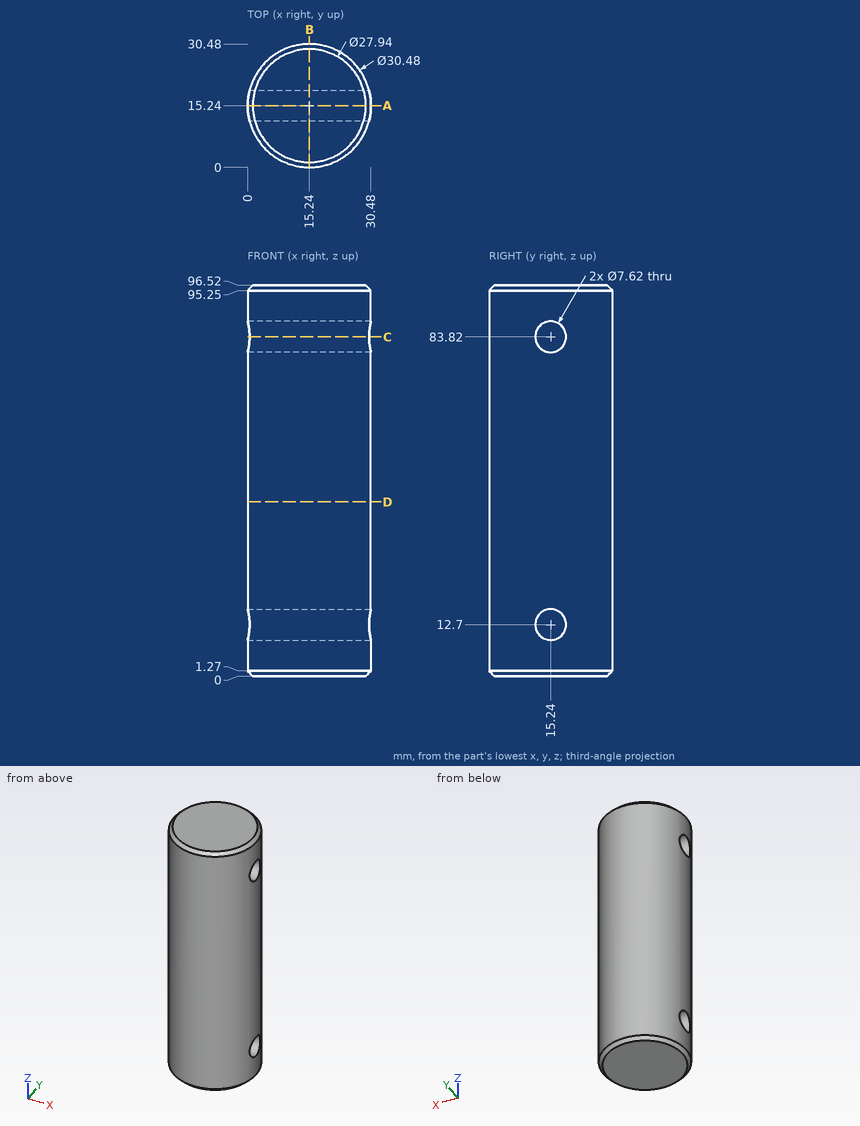
Source: three-view drawing plus pictorial views. Frame: mm from the lowest corner of the part. Coordinates: 2 decimals unless noted, no trailing zeros. Write each loop counter-clockwise with the first axis right and the second up, starting at its lowest first coordinate (ties: lowest second). Pieces come first, ordered by that corner, then holes. Notation, with made-up numbers: (62, 86.5) - (87, 86.5) arc R17 cw to (87, 102.5) - close; hole circle Ø9 at (33, -31). An arc over 180 degrees is marked (long way). Return JSON: item names as keys, results as strings.
Item 1: Pin query (flat end, axial travel): pin 1 Ø1.5 at (x, z) = (7.5, 31.5) entering from -Y; pin 2 Ø8 at (y, z) = (20, 22) entering from +X; pin 3 Ø10 at (y, z) = (15.24, 12.7) entering from -X; pin 4 Ø1.5 at (y, z) = (17, 9.5) entering from +X. Return the tip coordinate at first contact, or that it passes through.
Completed:
{"pin 1": "stops at y = 1.7", "pin 2": "stops at x = 30.46", "pin 3": "stops at x = 0", "pin 4": "stops at x = 30.44"}
Item 2: Section query D-D (z = 43). Output: boundary loops of the cut face in (x, y), and give its area (3 significant figures).
Completed:
{"outline": "circle Ø30.48 at (15.24, 15.24)", "area": "730 mm2"}
Item 3: Section query B-B (x = 15.24). Output: boundary loops of the cut face in (y, z).
Completed:
{"outline": "(0, 1.27) - (1.27, 0) - (29.21, 0) - (30.48, 1.27) - (30.48, 95.25) - (29.21, 96.52) - (1.27, 96.52) - (0, 95.25) - close; hole circle Ø7.62 at (15.24, 12.7); hole circle Ø7.62 at (15.24, 83.82)"}
Item 4: Line query: L1, parallel to Z at x = 19, y = 15; L2, parallel to Z at x = 28.5, y = 17.5; L3, parallel to X at y = 15, z = 29. Output: solid intervals per line, ascending.
Completed:
{"L1": "z = 0 to 8.9, 16.5 to 80.02, 87.62 to 96.52", "L2": "z = 0 to 9.63, 15.77 to 80.75, 86.89 to 96.52", "L3": "x = 0 to 30.48"}
Item 5: Section query A-A (y = 15.24). Output: boundary loops of the cut face in (x, z), and give its area (3 significant figures).
Completed:
{"outline": "(0, 1.27) - (1.27, 0) - (29.21, 0) - (30.48, 1.27) - (30.48, 8.89) - (0, 8.89) - close; (0, 16.51) - (30.48, 16.51) - (30.48, 80.01) - (0, 80.01) - close; (0, 87.63) - (30.48, 87.63) - (30.48, 95.25) - (29.21, 96.52) - (1.27, 96.52) - (0, 95.25) - close", "area": "2,470 mm2"}
Item 6: Section query C-C (z = 83.82). Output: boundary loops of the cut face in (x, y).
Completed:
{"outline": "(0.48, 11.43) arc R15.24 ccw to (30, 11.43) - close; (0.48, 19.05) - (30, 19.05) arc R15.24 ccw to start"}
